Here's how the part is built. I have some questions about the finished solid (model axes, mm). A direction names the side the tool comes from. Give positions to 0.01 mm unless a question says otherwise; leave off trailing zeros. Order: outer loops, then holes, each group sorted by start corner. A loop starts at its lowest first (then second) coordinate and runs counter-clockwise, first axis right, second up. Notation, with made-up numbers: (-1, 48.5) -> (34, 48.5) arc R22 cw to (34, 55.5) -> close; hole circle Ø3 at (44, 46.5). An arc over 180 degrees is marked (long way). Write each question's results on one line, items separated by ' | '. Start each with the question number.
Q1. For faces 1 (the face through (38, -1, 5)), 2 (the face through (44, -28, -5)), 3 (the face through (-32.1, -19, 0)), 4 (the face through (8, -16, 25)), which set-ups out of +Z, -Z, +X, -X, +Y, -Y let a thin tool reach every point of the face, with its end or its side?
Q2. Imagine slicing it at B-B, the plane z = 0. State how many separate pieces and enclosed holes the cut face has, then the cut area to 3 significant figures.
Q3. Imagine slicing it at C-C, the plane y = -18.5. Please give me the cut outline in (x, z), then the cut area to 3 significant figures.
Q4. Imagine slicing it at D-D, the plane z = -27.5. Please give me the cut outline in (x, y).
Q5. Thinking about a two-plate mould opening in Z: for faces 5 (the face through (-35.59, -33.52, 25.72)), 6 (the face through (-30, -19, 20)), 7 (the face through (-35.82, -33.52, -25.49)), which applies, pulls with the +Z half, pulls with the -Z half, needs draft (parallel to the pull), parting line crosses it, or undercut?
Q6. Imagine slicing it at A-A, the plane x = 38.5. Please give me the cut outline in (y, z).
Q7. I'm going to push flat-ended pins straight in: pin 1 (4 mm diameter, centred on y = -28.5, z = -3, fed in from -X); pin 2 (4 mm diameter, centred on y = 1, z = 16, fed in from +X); pin 3 (16 mm diameter, centred on x = 9, y = -22, fed in from -Z); pin 4 (2 mm diameter, centred on x = -0.5, z = -9, fed in from -Y). Where does each tip first touch, or does it pass through?
Q8. I need wall thicknesses on line 1 along X through (y, z) = (-0.5, 0); line 2 along X through (y, z) = (-26, 6.5); line 3 along Z through (x, y) = (-7.5, -30.5). Which ranges of each line are inside material? Lowest first, please. Write a range as [from, to].
```python
from build123d import *

# Parameters (mm, degrees)
SKETCH1_W           = 81
SKETCH1_H           = 50
SKETCH1_R           = 1.5
BOSS_EXTRUDE1_DEPTH = 35
FILLET1_R           = 10
FILLET2_R           = 3
CUT_EXTRUDE1_DEPTH  = 32
BOSS_EXTRUDE2_DEPTH = 15.3
SKETCH4_W           = 1
SKETCH4_H           = 24
CUT_EXTRUDE2_DEPTH  = 15.3
SKETCH5_W           = 10
SKETCH5_H           = 5
CUT_EXTRUDE3_DEPTH  = 16.3
SKETCH6_R           = 1.25
BOSS_EXTRUDE3_DEPTH = 3
SKETCH7_W           = 5
SKETCH7_H           = 10
CUT_EXTRUDE4_DEPTH  = 10


with BuildPart() as part:
    # Sketch1 → Boss-Extrude1 (new body)
    with BuildSketch(Plane(origin=(0, 0, 0), x_dir=(1, 0, 0), z_dir=(0, 1, 0))):
        with Locations((5.4, 0)):
            Rectangle(SKETCH1_W, SKETCH1_H)
        with Locations(Location((-23.9, 5, 0), (0, 0, 270))):
            Circle(SKETCH1_R, mode=Mode.SUBTRACT)
        with Locations(Location((-23.9, -5, 0), (0, 0, 90))):
            Circle(SKETCH1_R, mode=Mode.SUBTRACT)
        with Locations(Location((24.1, 5, 0), (0, 0, 90))):
            Circle(SKETCH1_R, mode=Mode.SUBTRACT)
        with Locations(Location((24.1, -5, 0), (0, 0, 270))):
            Circle(SKETCH1_R, mode=Mode.SUBTRACT)
        Polygon((-21.1, 3), (-26.1, 3), (-26.1, -3), (-21.1, -3), (-21.1, -11.1), (21.1, -11.1), (21.1, 11.1), (-21.1, 11.1), align=None, mode=Mode.SUBTRACT)
    extrude(amount=-BOSS_EXTRUDE1_DEPTH)

    # Fillet1
    fillet1_edges = [part.edges().sort_by_distance(p)[0] for p in [
        (-35.1, -17.5, 25),
        (-35.1, -17.5, -25),
    ]]
    fillet(fillet1_edges, radius=FILLET1_R)

    # Fillet2
    fillet2_edges = [part.edges().sort_by_distance(p)[0] for p in [
        (45.9, -17.5, 25),
        (45.9, -17.5, -25),
    ]]
    fillet(fillet2_edges, radius=FILLET2_R)

    # Sketch3 → Cut-Extrude1 (cut)
    with BuildSketch(Plane.XZ.offset(35)):
        with BuildLine():
            Line((42.9, 22), (-25.1, 22))
            ThreePointArc((-25.1, 22), (-30.049747468, 19.949747468), (-32.1, 15))
            Line((-32.1, 15), (-32.1, -15))
            ThreePointArc((-32.1, -15), (-30.049747468, -19.949747468), (-25.1, -22))
            Line((-25.1, -22), (42.9, -22))
            Line((42.9, -22), (42.9, 22))
        make_face()
    extrude(amount=-CUT_EXTRUDE1_DEPTH, mode=Mode.SUBTRACT)

    # Sketch2 → Boss-Extrude2 (add)
    with BuildSketch(Plane(origin=(0, 0, 0), x_dir=(1, 0, 0), z_dir=(0, 1, 0))):
        with BuildLine():
            Line((10.1, 15), (30, 15))
            Line((30, 15), (30, -15))
            Line((30, -15), (10.1, -15))
            ThreePointArc((10.1, -15), (-34.9, 0), (10.1, 15))
        make_face()
        with BuildLine():
            Line((8.539088915, 12), (27, 12))
            Line((27, 12), (27, -12))
            Line((27, -12), (8.539088915, -12))
            ThreePointArc((8.539088915, -12), (-31.9, 0), (8.539088915, 12))
        make_face(mode=Mode.SUBTRACT)
    extrude(amount=BOSS_EXTRUDE2_DEPTH)

    # Sketch4 → Cut-Extrude2 (cut)
    with BuildSketch(Plane(origin=(0, 15.3, 0), x_dir=(1, 0, 0), z_dir=(0, 1, 0))):
        with Locations((27.5, 0)):
            Rectangle(SKETCH4_W, SKETCH4_H)
    extrude(amount=-CUT_EXTRUDE2_DEPTH, mode=Mode.SUBTRACT)

    # Sketch5 → Cut-Extrude3 (cut)
    with BuildSketch(Plane(origin=(45.9, 0, 0), x_dir=(0, 0, -1), z_dir=(1, 0, 0))):
        with Locations((0, -27.5)):
            Rectangle(SKETCH5_W, SKETCH5_H)
    extrude(amount=-CUT_EXTRUDE3_DEPTH, mode=Mode.SUBTRACT)

    # Sketch6 → Boss-Extrude3 (add)
    with BuildSketch(Plane.XZ.offset(35)):
        with BuildLine():
            Line((42.9, 30), (-25.1, 30))
            ThreePointArc((-25.1, 30), (-35.706601718, 25.606601718), (-40.1, 15))
            Line((-40.1, 15), (-40.1, -15))
            ThreePointArc((-40.1, -15), (-35.706601718, -25.606601718), (-25.1, -30))
            Line((-25.1, -30), (42.9, -30))
            ThreePointArc((42.9, -30), (48.556854249, -27.656854249), (50.9, -22))
            Line((50.9, -22), (50.9, 22))
            ThreePointArc((50.9, 22), (48.556854249, 27.656854249), (42.9, 30))
        make_face()
        with Locations(Location((-25.1, 27.5, 0), (0, 0, 270))):
            Circle(SKETCH6_R, mode=Mode.SUBTRACT)
        with Locations(Location((42.9, 27.5, 0), (0, 0, 270))):
            Circle(SKETCH6_R, mode=Mode.SUBTRACT)
        with Locations(Location((42.9, -27.5, 0), (0, 0, 270))):
            Circle(SKETCH6_R, mode=Mode.SUBTRACT)
        with Locations(Location((-25.1, -27.5, 0), (0, 0, 270))):
            Circle(SKETCH6_R, mode=Mode.SUBTRACT)
        with BuildLine():
            Line((45.9, -22), (45.9, 22))
            ThreePointArc((45.9, 22), (45.021320344, 24.121320344), (42.9, 25))
            Line((42.9, 25), (-25.1, 25))
            ThreePointArc((-25.1, 25), (-32.171067812, 22.071067812), (-35.1, 15))
            Line((-35.1, 15), (-35.1, -15))
            ThreePointArc((-35.1, -15), (-32.171067812, -22.071067812), (-25.1, -25))
            Line((-25.1, -25), (42.9, -25))
            ThreePointArc((42.9, -25), (45.021320344, -24.121320344), (45.9, -22))
        make_face(mode=Mode.SUBTRACT)
    extrude(amount=-BOSS_EXTRUDE3_DEPTH)

    # Sketch7 → Cut-Extrude4 (cut)
    with BuildSketch(Plane(origin=(0, 0, 0), x_dir=(1, 0, 0), z_dir=(0, 1, 0))):
        with Locations((38.4, 0)):
            Rectangle(SKETCH7_W, SKETCH7_H)
    extrude(amount=-CUT_EXTRUDE4_DEPTH, mode=Mode.SUBTRACT)


solid = part.part
```
Geometry check:
1) face 1: +Y, -Y | face 2: +X | face 3: -Y | face 4: +Z, +X, -X, +Y
2) separate pieces: 4 | enclosed holes: 0 | area: 370 mm²
3) outline: (-35.1, -15) arc R10 ccw to (-25.1, -25) -> (42.9, -25) arc R3 ccw to (45.9, -22) -> (45.9, 22) arc R3 ccw to (42.9, 25) -> (-25.1, 25) arc R10 ccw to (-35.1, 15) -> close; hole (-32.1, -15) arc R7 ccw to (-25.1, -22) -> (42.9, -22) -> (42.9, 22) -> (-25.1, 22) arc R7 ccw to (-32.1, 15) -> close | area: 724 mm²
4) outline: (-33.39, -35) -> (-26.35, -35) -> (-26.35, -32) -> (-33.39, -32) -> close; (-23.85, -35) -> (41.65, -35) -> (41.65, -32) -> (-23.85, -32) -> close; (44.15, -35) -> (48.71, -35) -> (48.71, -32) -> (44.15, -32) -> close
5) face 5: pulls with the +Z half | face 6: undercut | face 7: pulls with the -Z half
6) outline: (-35, -30) -> (-32, -30) -> (-32, -25) -> (0, -25) -> (0, -5) -> (-3, -5) -> (-3, -22) -> (-35, -22) -> close; (-35, 22) -> (-3, 22) -> (-3, 5) -> (0, 5) -> (0, 25) -> (-32, 25) -> (-32, 30) -> (-35, 30) -> close
7) pin 1: x = -35.1 | pin 2: x = 45.9 | pin 3: z = -25 | pin 4: through
8) line 1: [-35.1, -26.1], [21.1, 35.9], [40.9, 45.9] | line 2: [-35.1, -32.1], [42.9, 45.9] | line 3: [-25, -22], [22, 25]
